Check sheet for the modelled part. Datum: model origin and axes. Units: mm. Round coordinates to 2 decimals unless told otherwise and drop trailing zeros. Write each loop counter-clockwise with the first axis right and the second up, starting at its lowest first coordinate (ties: lowest second). Pieces come first, ordered by that corner, then holes.
Item 1: Cross-section at B-B on x = 4. Enter the section's corners in (y, z).
Item 2: Material ranges on line 1 (Y direction, x = -5.25, z = -5); line 2 (X direction, y = 92.5, z = 2.75); line 3 (Y direction, x = 10, z = -8.25), recorded low to high.
Item 3: Cross-section at C-C on x = -3.25. Enter the section's corners in (y, z).
Item 4: Go/stop test with flat-tipped pins: pin 1 Ø12 at (x, z) = (0, 3) entering from -Y; pin 2 Ø5 at (x, z) = (-8, 5.5) entering from +Y; pin 3 Ø4 at (x, z) = (7, 9.5) entering from -Y. Record where each tip stops, or that it passes through.
from build123d import *

# Parameters (mm, degrees)
F0_W       = 25.4
F0_H       = 25.4
F1_DEPTH   = 101.6
F2_SIZE2   = 10.521014
F2_SIZE    = 25.39999
F2_2_SIZE2 = 10.521014
F2_2_SIZE  = 25.39999


# Not quite as in the source:
# - a fillet or chamfer is up to 0.001 mm smaller than in the source, because OpenCascade refuses the exact size


with BuildPart() as f1:
    # F0 (on Front) → F1 (new body, symmetric)
    with BuildSketch(Plane.XZ):
        Rectangle(F0_W, F0_H)
    extrude(amount=F1_DEPTH, both=True)

    # F2 (size 25.4 and 10.5210244843 in the source; OpenCascade refuses exactly that, so slightly less here)
    f2_edges = [f1.edges().sort_by_distance(p)[0] for p in [
        (12.7, -101.6, 0),
    ]]
    f2_side = f1.faces().sort_by_distance((0, -101.6, 0))[0]
    chamfer(f2_edges, length=F2_SIZE, length2=F2_SIZE2, reference=f2_side)

    # F2#2 (size 25.4 and 10.5210244843 in the source; OpenCascade refuses exactly that, so slightly less here)
    f2_2_edges = [f1.edges().sort_by_distance(p)[0] for p in [
        (12.7, 101.6, 0),
    ]]
    f2_2_side = f1.faces().sort_by_distance((0, 101.6, 0))[0]
    chamfer(f2_2_edges, length=F2_2_SIZE, length2=F2_2_SIZE2, reference=f2_2_side)


solid = f1.part
Response values:
1. outline: (-94.68, -12.7) - (94.68, -12.7) - (94.68, 12.7) - (-94.68, 12.7) - close
2. line 1: y = -98.51 to 98.51
2. line 2: x = -12.7 to 9.27
2. line 3: y = -92.2 to 92.2
3. outline: (-97.69, -12.7) - (97.69, -12.7) - (97.69, 12.7) - (-97.69, 12.7) - close
4. pin 1: stops at y = -98.82
4. pin 2: stops at y = 100.69
4. pin 3: stops at y = -94.27
